CAD build for the part. Positions are in the model's coordinates, mm. Round coordinates to 2 decimals unless told otherwise and drop trailing zeros. Loops run counter-clockwise (first coordinate to the right, second up) from the corner with the lowest first, then second, coordinate; pieces in that order, holes last. Notation, with made-up numbers: M -6.75,29.25 L 14.25,29.25 A25 cw 14.25,49.25 Z; hole C 0.25,-20.5 d2. An arc over 180 degrees is marked long. Use one line per item in the form item = value.
from build123d import *

# Parameters (mm, degrees)
SKETCH9_W           = 152.4
SKETCH9_H           = 203.2
BOSS_EXTRUDE4_DEPTH = 7.62
SKETCH10_R          = 14.605
CUT_EXTRUDE4_DEPTH  = 7.62
CUT_EXTRUDE5_DEPTH  = 7.62
FILLET2_R           = 25.4
CUT_EXTRUDE6_DEPTH  = 7.62


with BuildPart() as part:
    # Sketch9 → Boss-Extrude4 (new body)
    with BuildSketch(Plane(origin=(0, 0, 0), x_dir=(1, 0, 0), z_dir=(0, 1, 0))):
        with Locations((76.2, -101.6)):
            Rectangle(SKETCH9_W, SKETCH9_H)
    extrude(amount=BOSS_EXTRUDE4_DEPTH)

    # Sketch10 → Cut-Extrude4 (cut)
    with BuildSketch(Plane(origin=(0, 7.62, 0), x_dir=(1, 0, 0), z_dir=(0, 1, 0))):
        with Locations(Location((19.05, -41.770926028, 0), (0, 0, 270))):
            Circle(SKETCH10_R)
        with Locations(Location((133.35, -41.770926028, 0), (0, 0, 270))):
            Circle(SKETCH10_R)
    extrude(amount=-CUT_EXTRUDE4_DEPTH, mode=Mode.SUBTRACT)

    # Sketch11 → Cut-Extrude5 (cut)
    with BuildSketch(Plane(origin=(0, 7.62, 0), x_dir=(1, 0, 0), z_dir=(0, 1, 0))):
        Polygon((0, -101.6), (101.6, -203.2), (0, -203.2), align=None)
    extrude(amount=-CUT_EXTRUDE5_DEPTH, mode=Mode.SUBTRACT)

    # Fillet2
    fillet2_edges = [part.edges().sort_by_distance(p)[0] for p in [
        (101.6, 3.81, 203.2),
        (152.4, 3.81, 203.2),
    ]]
    fillet(fillet2_edges, radius=FILLET2_R)

    # Sketch12 → Cut-Extrude6 (cut)
    with BuildSketch(Plane(origin=(0, 7.62, 0), x_dir=(1, 0, 0), z_dir=(0, 1, 0))):
        Polygon((17.78, -3.670926028), (6.781477372, -22.720926028), (28.778522628, -22.720926028), align=None)
        Polygon((35.991477372, -22.720926028), (57.988522628, -22.720926028), (46.99, -3.670926028), align=None)
        Polygon((65.201477372, -22.720926028), (87.198522628, -22.720926028), (76.2, -3.670926028), align=None)
        Polygon((94.411477372, -22.720926028), (116.408522628, -22.720926028), (105.41, -3.670926028), align=None)
        Polygon((123.621477372, -22.720926028), (145.618522628, -22.720926028), (134.62, -3.670926028), align=None)
        Polygon((35.991477372, -48.120926028), (57.988522628, -48.120926028), (46.99, -29.070926028), align=None)
        Polygon((35.991477372, -73.520926028), (57.988522628, -73.520926028), (46.99, -54.470926028), align=None)
        Polygon((35.991477372, -98.920926028), (57.988522628, -98.920926028), (46.99, -79.870926028), align=None)
        Polygon((35.991477372, -124.320926028), (57.988522628, -124.320926028), (46.99, -105.270926028), align=None)
        Polygon((65.201477372, -48.120926028), (87.198522628, -48.120926028), (76.2, -29.070926028), align=None)
        Polygon((105.41, -29.070926028), (94.411477372, -48.120926028), (116.408522628, -48.120926028), align=None)
        Polygon((65.201477372, -73.520926028), (87.198522628, -73.520926028), (76.2, -54.470926028), align=None)
        Polygon((105.41, -54.470926028), (94.411477372, -73.520926028), (116.408522628, -73.520926028), align=None)
        Polygon((65.201477372, -98.920926028), (87.198522628, -98.920926028), (76.2, -79.870926028), align=None)
        Polygon((105.41, -79.870926028), (94.411477372, -98.920926028), (116.408522628, -98.920926028), align=None)
        Polygon((65.201477372, -124.320926028), (87.198522628, -124.320926028), (76.2, -105.270926028), align=None)
        Polygon((105.41, -105.270926028), (94.411477372, -124.320926028), (116.408522628, -124.320926028), align=None)
        Polygon((65.201477372, -149.720926028), (87.198522628, -149.720926028), (76.2, -130.670926028), align=None)
        Polygon((105.41, -130.670926028), (94.411477372, -149.720926028), (116.408522628, -149.720926028), align=None)
        Polygon((130.81, -79.870926028), (119.811477372, -98.920926028), (141.808522628, -98.920926028), align=None)
        Polygon((130.81, -105.270926028), (119.811477372, -124.320926028), (141.808522628, -124.320926028), align=None)
        Polygon((130.81, -130.670926028), (119.811477372, -149.720926028), (141.808522628, -149.720926028), align=None)
        Polygon((105.41, -156.070926028), (94.411477372, -175.120926028), (116.408522628, -175.120926028), align=None)
        Polygon((130.81, -156.070926028), (119.811477372, -175.120926028), (141.808522628, -175.120926028), align=None)
        Polygon((10.591477372, -98.920926028), (32.588522628, -98.920926028), (21.59, -79.870926028), align=None)
    extrude(amount=-CUT_EXTRUDE6_DEPTH, mode=Mode.SUBTRACT)


solid = part.part
1. Cut at A-A on x = 137.5. Write the cut outline in (y, z).
Completed:
outline = M 0,0 L 7.62,0 L 7.62,8.66 L 0,8.66 Z; M 0,22.72 L 7.62,22.72 L 7.62,27.77 L 0,27.77 Z; M 0,55.77 L 7.62,55.77 L 7.62,91.46 L 0,91.46 Z; M 0,98.92 L 7.62,98.92 L 7.62,116.86 L 0,116.86 Z; M 0,124.32 L 7.62,124.32 L 7.62,142.26 L 0,142.26 Z; M 0,149.72 L 7.62,149.72 L 7.62,167.66 L 0,167.66 Z; M 0,175.12 L 7.62,175.12 L 7.62,200.93 L 0,200.93 Z
2. Drop flat-ended pins along their axis: P1, Ø4, axis at x = 134.5, y = 4, coming from the -Z side; P2, Ø17.5, axis at x = 19.05, z = 41.77, coming from the +Y side; P3, Ø1, axis at y = 4, z = 123, coming from the -X side. Give the stop position or say it passes through.
Completed:
P1 = 0
P2 = through
P3 = 20.9
3. Cut at D-D on y = 3.5. State how many separate pieces and enclosed holes the cut face has, and give its area (3 significant figures).
Completed:
separate_pieces = 1
enclosed_holes = 27
area = 19,100 mm2
4. Probe line 1 along Z through (x, y) = (145, 6.25); line 2 along X through (y, z) = (1.25, 133); line 3 along X through (y, z) = (1.75, 35). List the from-to ranges inside material, lowest first. Write a range as from..to.
Completed:
line_1 = 0..21.65, 22.72..32.96, 50.58..195.72
line_2 = 31.4..74.86, 77.54..104.07, 106.75..129.47, 132.15..152.4
line_3 = 0..6.11, 31.99..43.57, 50.41..72.78, 79.62..101.99, 108.83..120.41, 146.29..152.4
5. Cut at B-B on x = 39.5. Write the cut outline in (y, z), and give its area (3 significant figures).
Completed:
outline = M 0,0 L 7.62,0 L 7.62,16.64 L 0,16.64 Z; M 0,22.72 L 7.62,22.72 L 7.62,42.04 L 0,42.04 Z; M 0,48.12 L 7.62,48.12 L 7.62,67.44 L 0,67.44 Z; M 0,73.52 L 7.62,73.52 L 7.62,92.84 L 0,92.84 Z; M 0,98.92 L 7.62,98.92 L 7.62,118.24 L 0,118.24 Z; M 0,124.32 L 7.62,124.32 L 7.62,141.1 L 0,141.1 Z
area = 844 mm2
6. Cut at C-C on x = 14. Write the cut outline in (y, z), and give its area (3 significant figures).
Completed:
outline = M 0,0 L 7.62,0 L 7.62,10.22 L 0,10.22 Z; M 0,22.72 L 7.62,22.72 L 7.62,28.07 L 0,28.07 Z; M 0,55.48 L 7.62,55.48 L 7.62,93.02 L 0,93.02 Z; M 0,98.92 L 7.62,98.92 L 7.62,115.6 L 0,115.6 Z
area = 532 mm2
7. Pull direction X, two halves, no side cores. Call faces 1 (the face through (140.196, 3.863, 13.329)), 2 (the face through (70.78, 3.86, 38.46)): +X half, -X half, draft (parallel to the pull), parting line (faces both ways), or undercut.
Completed:
face_1 = undercut
face_2 = undercut
